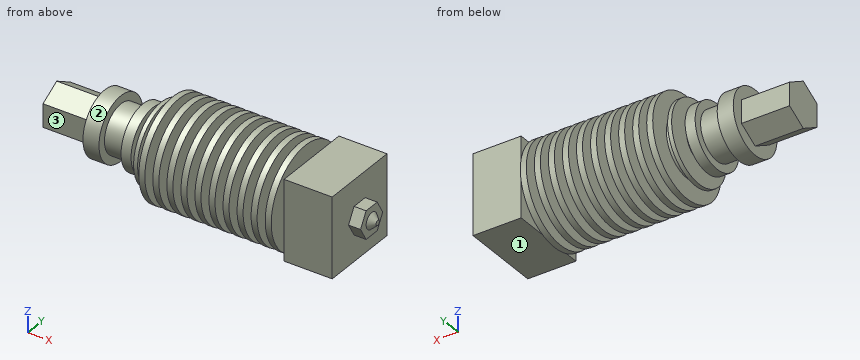
from build123d import *

# Parameters (mm, degrees)
SKETCH_2_R      = 3
EXTRUDE_1_DEPTH = 1.5
SKETCH_3_W      = 20
SKETCH_3_H      = 20
EXTRUDE_2_DEPTH = 12
EXTRUDE_3_DEPTH = 3
EXTRUDE_4_DEPTH = 12


with BuildPart() as part:
    # 草圖1 → 旋轉1 (revolve)
    with BuildSketch(Plane.XY):
        Polygon((0, 0), (-50, 0), (-50, 8), (-46, 8), (-46, 6), (-40.5, 6), (-40.5, 8), (-38, 8), (-38, 4.5), (-36, 4.5), (-36, 10), (-35, 10), (-35, 7.5), (-33, 7.5), (-33, 12.5), (-31.5, 12.5), (-31.5, 7.5), (-29.5, 7.5), (-29.5, 12.5), (-28, 12.5), (-28, 7.5), (-26, 7.5), (-26, 12.5), (-24.5, 12.5), (-24.5, 7.5), (-22.5, 7.5), (-22.5, 12.5), (-21, 12.5), (-21, 7.5), (-19, 7.5), (-19, 12.5), (-17.5, 12.5), (-17.5, 7.5), (-15.5, 7.5), (-15.5, 12.5), (-14, 12.5), (-14, 7.5), (-12, 7.5), (-12, 12.5), (-10.5, 12.5), (-10.5, 7.5), (-8.5, 7.5), (-8.5, 12.5), (-7, 12.5), (-7, 7.5), (-5, 7.5), (-5, 12.5), (-3.5, 12.5), (-3.5, 7.5), (-1.5, 7.5), (-1.5, 12.5), (0, 12.5), align=None)
    revolve(axis=Axis((0, 0, 0), (-1, 0, 0)))

    # 草圖2 → 填料-伸長1 (add)
    with BuildSketch(Plane(origin=(0, 0, 0), x_dir=(0, 0, -1), z_dir=(1, 0, 0))):
        with Locations(Location((0, 0, 0), (0, 0, 90))):
            Circle(SKETCH_2_R)
    extrude(amount=EXTRUDE_1_DEPTH)

    # 草圖3 → 填料-伸長2 (add)
    with BuildSketch(Plane(origin=(1.5, 0, 0), x_dir=(0, 0, -1), z_dir=(1, 0, 0))):
        Rectangle(SKETCH_3_W, SKETCH_3_H)
    extrude(amount=EXTRUDE_2_DEPTH)

    # 草圖4 → 填料-伸長3 (add)
    with BuildSketch(Plane(origin=(13.5, 0, 0), x_dir=(0, 0, -1), z_dir=(1, 0, 0))):
        Polygon((0, 4.041451884), (-3.5, 2.020725942), (-3.5, -2.020725942), (0, -4.041451884), (3.5, -2.020725942), (3.5, 2.020725942), align=None)
    extrude(amount=EXTRUDE_3_DEPTH)

    # 草圖6 → 旋轉2 (revolve)
    with BuildSketch(Plane.XY, mode=Mode.PRIVATE) as revolve_2_sk:
        Polygon((16.5, 0), (18, 0), (18, 0.6), (16.5, 2), align=None)
    revolve(revolve_2_sk.sketch.rotate(Axis((16.5, 0, 0), (1, 0, 0)), 180), axis=Axis((16.5, 0, 0), (1, 0, 0)))

    # 草圖7 → 填料-伸長4 (add)
    with BuildSketch(Plane.ZY.offset(50)):
        Polygon((-5.773502692, 0), (-2.886751346, -5), (2.886751346, -5), (5.773502692, 0), (2.886751346, 5), (-2.886751346, 5), align=None)
    extrude(amount=EXTRUDE_4_DEPTH)


solid = part.part
CAD build for the part. Positions are in the model's coordinates, mm. Face numbers are marked on the shaded views. A direction names the side the tool comes from. Coordinates: 2 decimals unless noted, no trailing zeros.
Item 1: Drill centre lines: L1, parallel to X at y = 3, z = 4; L2, parallel to X at y = 2, z = -3.75; L3, parallel to Y at x = 10, z = 5.25. Where is each one in solid material? Low to high.
Check sheet entries:
L1: x = -62 to -38, -36 to 0, 1.5 to 13.5
L2: x = -62 to 0, 1.5 to 13.5
L3: y = -10 to 10
Item 2: 3-axis set-ups, long thin cutter, end or side, ignore diameter. For the marked faces 1, 2 and 3: which of +Z, -Z, +X, -X, +Y, -Y reach the whole face in a straight line?
Check sheet entries:
face 1: -Z, +X, +Y, -Y
face 2: -X
face 3: +Z, -Z, -X, -Y
Item 3: Pin check, flat tips, straight feed: pin 1 Ø10 at (y, z) = (6, -8.5) entering from -X; pin 2 Ø8 at (y, z) = (8.5, -7) entering from +X; pin 3 Ø13 at (x, z) = (7.5, 0) entering from +Y. Stop position of each tip, or through.
Check sheet entries:
pin 1: stops at x = -50
pin 2: stops at x = 13.5
pin 3: stops at y = 10
